Geometry: final body of the model. Coordinates: model frame, mm. A direction names the side the tool comes from. Give positions to 0.01 mm unless a question says otherwise; leave off trailing zeros. Write each loop counter-clockwise with the first axis right and the second up, starting at its lowest first coordinate (ties: lowest second). Pieces come first, ordered by that corner, then holes. Notation, with made-up numbers: M 37.5,26.5 L 66.5,26.5 A25 cw 66.5,65.5 Z; hole C 77.5,-24.75 d2. An arc over 180 degrees is marked long. Use a Markdown table: item, result. Add a question column.
(1) Pin query (flat end, axial travel): pin 1 Ø3.5 at (x, z) = (22.5, 5.3) entering from -Y; pin 2 Ø2 at (x, y) = (-16.5, -1.5) entering from +Z; pin 3 Ø1.5 at (x, y) = (-12, 2.5) entering from +Z; pin 4 Ø1 at (x, y) = (5.5, -4.5) entering from -Z. Return the tip coordinate at first contact, or that it passes through.
(2) Cut plane A-A (x = -22.5). Output: boundary loops of the cut face in (y, z).
(3) Cut plane B-B (x = -5.8). Output: boundary loops of the cut face in (y, z), plus the area to 3 significant figures.
(4) Cut plane D-D (y = -3.75). Output: boundary loops of the cut face in (x, z), plus the area to 3 significant figures.
(5) Cut plane C-C (y = 3). Output: boundary loops of the cut face in (x, z).
(6) Material intervals for L1, parallel to X at y = 2.75, z = 8.25; L2, parallel to Z at x = 22.5, y = 3.8; L3, parallel to Y at x = -17.5, z = 9.5, sorted ascending.
(7) Draft query along X for faces 5 (the flat face through (-30, 3, 4)), 6 (the cylindrical face through (-24, 3.04, 5.23)), 7 (the flat face through (30, 3, 4)), 8 (the cylindrical face through (-32.47, 1.99, 5.19)). Return one class per face: released by +X, released by -X, zero draft, split by the parting line, or undercut.
(8) Reachability of faces 1 (the flat face through (-35, 3, 6)), 2 (the cylindrical face through (32.465, 1.735, 5.493)), 3 (the cylindrical face through (5.585, -2.958, 1.163)), 4 (the flat face through (0, 3, 5.299)) from +Z, -Z, +X, -X, +Y, -Y: full face, straight path, thin tool, end or side. Return the list, or none.
Autodesk Inventor part; units mm, degrees
ref_plane "YZ Plane" through (0, 0, 0) normal (1, 0, 0) x (0, 1, 0)
ref_plane "XZ Plane" through (0, 0, 0) normal (0, 1, 0) x (-1, 0, 0)
ref_plane "XY Plane" through (0, 0, 0) normal (0, 0, 1) x (1, 0, 0)
sketch "Skizze1" plane through (0, 0, 0) normal (0, 1, 0) x (-1, 0, 0)
  line L0 (30, 0.2989) -> (30, 10.2989)
  line L1 (30, 10.2989) -> (15, 10.2989)
  line L2 (15, 10.2989) -> (15, 5.2989)
  line L3 (15, 5.2989) -> (-15, 5.2989)
  line L4 (-15, 5.2989) -> (-15, 10.2989)
  line L5 (-15, 10.2989) -> (-30, 10.2989)
  line L6 (-30, 10.2989) -> (-30, 0.2989)
  line L7 (-30, 0.2989) -> (30, 0.2989)
  line L8 (0, -2.0598) -> (0, 12.3587)
  point P0 (0, 0)
  dimension "d0" = 30
  dimension "d1" = 5
  dimension "d2" = 15
  dimension "d3" = 15
  dimension "d4" = 15
  dimension "d5" = 5
extrude "Extrusion1" add sketch "Skizze1" along normal blind 6
sketch "Skizze2" plane through (30, 0, 10.2989) normal (1, 0, 0) x (0, 0, -1)
  circle A0 centre (4, 3) radius 1.5
  line L0 (0, 0) -> (0, 6)
  line L1 (0, 6) -> (10, 6)
  point P0 (10.2989, 0)
  dimension "d8" = 3
  dimension "d9" = 4
  dimension "d10" = 3
extrude "Extrusion2" add sketch "Skizze2" along normal blind 5
sketch "Skizze4" plane through (-30, 0, 0.2989) normal (-1, 0, 0) x (0, 0, 1)
  circle A0 centre (6, 3) radius 1.5
  circle A1 centre (6, 3) radius 1.5
  line L0 (10, 0) -> (10, 6)
  line L1 (0, 0) -> (10, 0)
  point P0 (-0.2989, 0)
  dimension "d21" = 4
  dimension "d22" = 3
extrude "Extrusion4" add sketch "Skizze4" along normal blind 5
sketch "Skizze5" plane through (0, 6, 0) normal (0, 1, 0) x (1, 0, 0)
  circle A0 centre (-22.5, -5.2989) radius 1.5
  circle A1 centre (22.5, -5.2989) radius 1.5
  line L0 (-30, -10.2989) -> (-15, -10.2989)
  line L1 (-30, -0.2989) -> (-30, -10.2989)
  line L2 (30, -10.2989) -> (30, -0.2989)
  line L3 (15, -10.2989) -> (30, -10.2989)
  point P0 (0, 0)
  dimension "d25" = 5
  dimension "d26" = 7.5
  dimension "d27" = 7.5
  dimension "d28" = 5
  dimension "d29" = 3
  dimension "d30" = 3
extrude "Extrusion5" cut sketch "Skizze5" against normal blind 6
sketch "Skizze6" plane through (0, 0, 0) normal (0, -1, 0) x (1, 0, 0)
  circle A0 centre (-5.8, 2.7989) radius 1.65
  circle A1 centre (5.8, 2.7989) radius 1.65
  line L0 (-30, 0.2989) -> (-30, 10.2989)
  line L1 (-30, 10.2989) -> (-15, 10.2989)
  line L2 (15, 10.2989) -> (30, 10.2989)
  line L3 (30, 10.2989) -> (30, 0.2989)
  point P0 (0, 0)
  dimension "d33" = 3.3
  dimension "d34" = 3.3
  dimension "d36" = 7.5
  dimension "d37" = 7.5
  dimension "d41" = 5.8
  dimension "d42" = 5.8
extrude "Extrusion6" add sketch "Skizze6" along normal blind 6
equation "\"d2\" = 0.5 * d0"
properties part number "Fuehrungslagerhalter_v1"
Answer list:
| question | item | result |
|---|---|---|
| 1 | pin 1 | y = 0 |
| 1 | pin 2 | through |
| 1 | pin 3 | z = 5.3 |
| 1 | pin 4 | z = 1.15 |
| 2 | outline | M 0,0.3 L 6,0.3 L 6,3.8 L 0,3.8 Z; M 0,6.8 L 6,6.8 L 6,10.3 L 0,10.3 Z |
| 3 | outline | M -6,1.15 L 0,1.15 L 0,0.3 L 6,0.3 L 6,5.3 L 0,5.3 L 0,4.45 L -6,4.45 Z |
| 3 | area | 49.8 mm² |
| 4 | outline | C -5.8,2.8 d3.3; C 5.8,2.8 d3.3 |
| 4 | area | 17.1 mm² |
| 5 | outline | M -35,4.8 L -30,4.8 L -30,0.3 L 30,0.3 L 30,4.8 L 35,4.8 L 35,7.8 L 30,7.8 L 30,10.3 L 15,10.3 L 15,5.3 L -15,5.3 L -15,10.3 L -30,10.3 L -30,7.8 L -35,7.8 Z; hole C -22.5,5.3 d3; hole C 22.5,5.3 d3 |
| 6 | L1 | -30 to -15, 15 to 30 |
| 6 | L2 | 0.3 to 3.8, 6.8 to 10.3 |
| 6 | L3 | 0 to 6 |
| 7 | face 5 | released by -X |
| 7 | face 6 | undercut |
| 7 | face 7 | released by +X |
| 7 | face 8 | zero draft |
| 8 | face 1 | +Z, -Z, -X, +Y, -Y |
| 8 | face 2 | +X |
| 8 | face 3 | -Y |
| 8 | face 4 | +Z, +Y, -Y |
